from build123d import *

# Parameters (mm, degrees)
SKETCH_1_W      = 13
SKETCH_1_H      = 27
EXTRUDE_1_DEPTH = 1.6
SKETCH_2_W      = 8.033918408
SKETCH_2_H      = 5.268143219
SKETCH_2_W_2    = 8.560732729
SKETCH_2_H_2    = 8.56073273
SKETCH_2_W_3    = 1.185332224
SKETCH_2_H_3    = 2.546269222
EXTRUDE_2_DEPTH = 1


with BuildPart() as part:
    # 草图1 → 凸台-拉伸1 (new body)
    with BuildSketch(Plane(origin=(0, 0, 0), x_dir=(1, 0, 0), z_dir=(0, 1, 0))):
        Rectangle(SKETCH_1_W, SKETCH_1_H)
    extrude(amount=EXTRUDE_1_DEPTH)

    # 草图2 → 凸台-拉伸2 (add)
    with BuildSketch(Plane(origin=(0, 1.6, 0), x_dir=(1, 0, 0), z_dir=(0, 1, 0))):
        with Locations((1.853625196, -10.38263226)):
            Rectangle(SKETCH_2_W, SKETCH_2_H)
        with Locations((-0.165829704, -1.229233418)):
            Rectangle(SKETCH_2_W_2, SKETCH_2_H_2)
        with Locations((-5.346170536, 2.392615045)):
            Rectangle(SKETCH_2_W_3, SKETCH_2_H_3)
    extrude(amount=EXTRUDE_2_DEPTH)


solid = part.part
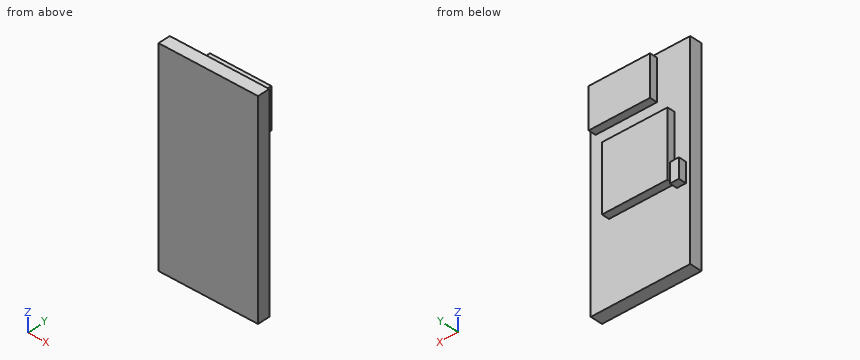
Design review of the part built by this model. Coordinates are the model's own, in mm. Coordinates: 2 decimals unless noted, no trailing zeros. Loops run counter-clockwise (first coordinate to the right, second up) from the corner with the lowest first, then second, coordinate; pieces in that order, holes last. Notation, with made-up numbers: M 85,-32.75 L 97,-32.75 A14 ccw 97,-16.75 Z; hole C -10,-39 d9. An arc over 180 degrees is marked long. Use one line per item in the form item = value.
(1) For line 1 along Z through (x, y) = (-1, 2.15); line 2 along X through (y, z) = (2.15, -2); line 3 along Y through (x, z) = (-4.75, 8.5), list the stretches that pass through material, from the lowest coordinate up. Write a range as from..to.
Return value:
line_1 = -3.05..5.51, 7.75..13.02
line_2 = -5.94..-4.75, -4.45..4.11
line_3 = 0..1.6
(2) Consider section B-B (x = 2.5). Write out the cut boundary in (y, z), and give its area (3 significant figures).
Return value:
outline = M 0,-13.5 L 1.6,-13.5 L 1.6,-3.05 L 2.6,-3.05 L 2.6,5.51 L 1.6,5.51 L 1.6,7.75 L 2.6,7.75 L 2.6,13.02 L 1.6,13.02 L 1.6,13.5 L 0,13.5 Z
area = 57.0 mm2
(3) Consider section A-A (y = 2). Write out the cut boundary in (x, z), and give its area (3 significant figures).
Return value:
outline = M -5.94,-3.67 L -4.75,-3.67 L -4.75,-1.12 L -5.94,-1.12 Z; M -4.45,-3.05 L 4.11,-3.05 L 4.11,5.51 L -4.45,5.51 Z; M -2.16,7.75 L 5.87,7.75 L 5.87,13.02 L -2.16,13.02 Z
area = 119 mm2
(4) Clearance check with flat-ended pins moving along their axes: P1, Ø0.5, axis at y = 2, z = 10.5, coming from the -X side; P2, Ø0.5, axis at x = 0, y = 2, coming from the +Z side; P3, Ø1.1, axis at x = -5.5, y = 2.5, coming from the -Z side. State where each tip first meets the part, or that it passes through.
Return value:
P1 = -2.16
P2 = 13.02
P3 = -3.67
(5) Consider section C-C (z = -2.25). Write out the cut boundary in (x, y), and give its area (3 significant figures).
Return value:
outline = M -6.5,0 L 6.5,0 L 6.5,1.6 L 4.11,1.6 L 4.11,2.6 L -4.45,2.6 L -4.45,1.6 L -4.75,1.6 L -4.75,2.6 L -5.94,2.6 L -5.94,1.6 L -6.5,1.6 Z
area = 30.5 mm2
(6) Consider section D-D (x = -5). Write out the cut boundary in (y, z), and give its area (3 significant figures).
Return value:
outline = M 0,-13.5 L 1.6,-13.5 L 1.6,-3.67 L 2.6,-3.67 L 2.6,-1.12 L 1.6,-1.12 L 1.6,13.5 L 0,13.5 Z
area = 45.7 mm2
